```python
from build123d import *

# Parameters (mm, degrees)
SKETCH001_R  = 20
PAD_DEPTH    = 5
POCKET_DEPTH = 2.5


with BuildPart() as part:
    # Sketch001 (on DatumPlane) → Pad (new body)
    with BuildSketch(Plane.XY):
        Circle(SKETCH001_R)
    extrude(amount=-PAD_DEPTH)

    # Sketch (on DatumPlane) → Pocket (cut)
    with BuildSketch(Plane(origin=(-14.5, 14.5, 0), x_dir=(1, 0, 0), z_dir=(0, 0, 1))):
        with BuildLine():
            add(Edge.make_bspline(
                [(19.881144, 0), (19.819056, -0.000794), (19.75485, -0.003847), (19.69135, -0.008819)],
                knots=[0, 0, 0, 0, 1, 1, 1, 1], degree=3))
            add(Edge.make_bspline(
                [(19.69135, -0.008819), (17.16405, -0.4451), (15.774106, -3.117779), (15.573022, -5.474688)],
                knots=[0, 0, 0, 0, 1, 1, 1, 1], degree=3))
            add(Edge.make_bspline(
                [(15.573022, -5.474688), (15.278806, -7.61365), (16.221428, -10.361789), (18.569517, -10.841567)],
                knots=[0, 0, 0, 0, 1, 1, 1, 1], degree=3))
            add(Edge.make_bspline(
                [(18.569517, -10.841567), (18.9103, -10.906478), (19.263783, -10.876844), (19.596806, -10.786533)],
                knots=[0, 0, 0, 0, 1, 1, 1, 1], degree=3))
            add(Edge.make_bspline(
                [(19.596806, -10.786533), (22.424672, -9.838267), (23.689733, -6.489136), (23.281217, -3.715456)],
                knots=[0, 0, 0, 0, 1, 1, 1, 1], degree=3))
            add(Edge.make_bspline(
                [(23.281217, -3.715456), (23.161978, -1.923627), (21.811544, 0.024624), (19.881144, 0)],
                knots=[0, 0, 0, 0, 1, 1, 1, 1], degree=3))
        make_face()
        with BuildLine():
            add(Edge.make_bspline(
                [(9.165872, -0.114653), (7.593894, -0.153233), (6.369756, -1.747167), (6.120694, -3.245556)],
                knots=[0, 0, 0, 0, 1, 1, 1, 1], degree=3))
            add(Edge.make_bspline(
                [(6.120694, -3.245556), (5.595691, -6.21411), (6.946053, -9.902472), (10.038644, -10.841567)],
                knots=[0, 0, 0, 0, 1, 1, 1, 1], degree=3))
            add(Edge.make_bspline(
                [(10.038644, -10.841567), (10.328628, -10.904361), (10.627783, -10.910711), (10.920589, -10.865556)],
                knots=[0, 0, 0, 0, 1, 1, 1, 1], degree=3))
            add(Edge.make_bspline(
                [(10.920589, -10.865556), (13.01115, -10.517011), (13.896622, -8.173861), (13.809133, -6.281632)],
                knots=[0, 0, 0, 0, 1, 1, 1, 1], degree=3))
            add(Edge.make_bspline(
                [(13.809133, -6.281632), (13.746339, -3.785941), (12.449528, -0.900148), (9.858022, -0.198473)],
                knots=[0, 0, 0, 0, 1, 1, 1, 1], degree=3))
            add(Edge.make_bspline(
                [(9.858022, -0.198473), (9.620956, -0.135615), (9.390239, -0.109142), (9.165872, -0.114653)],
                knots=[0, 0, 0, 0, 1, 1, 1, 1], degree=3))
        make_face()
        with BuildLine():
            add(Edge.make_bspline(
                [(26.729267, -8.546042), (24.010761, -8.709025), (22.146683, -11.421886), (21.880689, -13.954831)],
                knots=[0, 0, 0, 0, 1, 1, 1, 1], degree=3))
            add(Edge.make_bspline(
                [(21.880689, -13.954831), (21.521561, -15.781514), (22.495228, -18.225558), (24.580144, -18.371608)],
                knots=[0, 0, 0, 0, 1, 1, 1, 1], degree=3))
            add(Edge.make_bspline(
                [(24.580144, -18.371608), (27.486328, -18.335625), (29.469644, -15.229769), (29.551489, -12.557125)],
                knots=[0, 0, 0, 0, 1, 1, 1, 1], degree=3))
            add(Edge.make_bspline(
                [(29.551489, -12.557125), (29.735639, -10.789708), (28.694239, -8.644114), (26.729267, -8.546042)],
                knots=[0, 0, 0, 0, 1, 1, 1, 1], degree=3))
        make_face()
        with BuildLine():
            add(Edge.make_bspline(
                [(2.932289, -9.148586), (1.775601, -9.138708), (0.638034, -9.831564), (0.260068, -11.007019)],
                knots=[0, 0, 0, 0, 1, 1, 1, 1], degree=3))
            add(Edge.make_bspline(
                [(0.260068, -11.007019), (-0.748383, -14.152386), (1.276632, -18.135953), (4.607983, -18.797058)],
                knots=[0, 0, 0, 0, 1, 1, 1, 1], degree=3))
            add(Edge.make_bspline(
                [(4.607983, -18.797058), (5.998351, -19.034831), (7.219809, -17.967325), (7.564826, -16.682508)],
                knots=[0, 0, 0, 0, 1, 1, 1, 1], degree=3))
            add(Edge.make_bspline(
                [(7.564826, -16.682508), (8.295076, -13.934369), (6.794712, -10.743847), (4.255206, -9.496425)],
                knots=[0, 0, 0, 0, 1, 1, 1, 1], degree=3))
            add(Edge.make_bspline(
                [(4.255206, -9.496425), (3.841538, -9.264297), (3.384973, -9.152114), (2.932289, -9.148586)],
                knots=[0, 0, 0, 0, 1, 1, 1, 1], degree=3))
        make_face()
        with BuildLine():
            add(Edge.make_bspline(
                [(15.120761, -14.788092), (12.853106, -14.793031), (10.550172, -15.943792), (9.081911, -17.656881)],
                knots=[0, 0, 0, 0, 1, 1, 1, 1], degree=3))
            add(Edge.make_bspline(
                [(9.081911, -17.656881), (7.495822, -19.653603), (6.196753, -21.976997), (5.688542, -24.496536)],
                knots=[0, 0, 0, 0, 1, 1, 1, 1], degree=3))
            add(Edge.make_bspline(
                [(5.688542, -24.496536), (5.07111, -26.309814), (6.470509, -28.397553), (8.409517, -28.410253)],
                knots=[0, 0, 0, 0, 1, 1, 1, 1], degree=3))
            add(Edge.make_bspline(
                [(8.409517, -28.410253), (10.742083, -28.474458), (12.746567, -26.872847), (15.065728, -26.754314)],
                knots=[0, 0, 0, 0, 1, 1, 1, 1], degree=3))
            add(Edge.make_bspline(
                [(15.065728, -26.754314), (17.033522, -26.454453), (18.795294, -27.477508), (20.564828, -28.147786)],
                knots=[0, 0, 0, 0, 1, 1, 1, 1], degree=3))
            add(Edge.make_bspline(
                [(20.564828, -28.147786), (22.071189, -28.791958), (24.152578, -28.545014), (24.921633, -26.923647)],
                knots=[0, 0, 0, 0, 1, 1, 1, 1], degree=3))
            add(Edge.make_bspline(
                [(24.921633, -26.923647), (25.526294, -25.271942), (24.635883, -23.509464), (23.898578, -22.042614)],
                knots=[0, 0, 0, 0, 1, 1, 1, 1], degree=3))
            add(Edge.make_bspline(
                [(23.898578, -22.042614), (22.394333, -19.660658), (20.782139, -17.157347), (18.315517, -15.670036)],
                knots=[0, 0, 0, 0, 1, 1, 1, 1], degree=3))
            add(Edge.make_bspline(
                [(18.315517, -15.670036), (17.327033, -15.057614), (16.228483, -14.785975), (15.120761, -14.788092)],
                knots=[0, 0, 0, 0, 1, 1, 1, 1], degree=3))
        make_face()
    extrude(amount=-POCKET_DEPTH, mode=Mode.SUBTRACT)


solid = part.part
```
Model file for the job. Use its own axes, mm. A direction names the side the tool comes from. Give positions to 0.01 mm unless a question says otherwise; leave off trailing zeros. Order: outer loops, then holes, each group sorted by start corner. A loop starts at its lowest first (then second) coordinate and runs counter-clockwise, first axis right, second up.
1) Saw through at D-D, the plane y = 15. Write the cut outline in (x, z).
2) Saw through at B-B, the plane z = -1.35. Count the separate pieces of the cut face and the enclosed holes in it, then the cut area to 3 significant figures.
3) Mould opens along Y. For faces 3 (the flat face through (0, 0, -5)), 4 (the cylindrical face through (-4.336, -19.524, -2.465)), 5 (the flat face through (5, 9, -2.5)) say: +Y half, -Y half, draft (parallel to the pull), parting line (faces both ways), or undercut.
4) 3-axis set-ups, long thin cutter, end or side, ignore diameter. For faces 1 (the flat face through (1, -7, -2.5)), 2 (the flat face through (0, 0, 0)): which of +Z, -Z, +X, -X, +Y, -Y reach the whole face in a straight line?
5) Saw through at C-C, the plane x = 17.5. Write the cut outline in (y, z), then the cut area to 3 significant figures.
6) Saw through at A-A, the plane z = -3.8. Write the cut outline in (x, y).
7) Wall check: probe 1 along X at (y, z) = (13, -1.95); probe 2 along X at (y, z) = (8.5, -2); probe 3 along X at (y, z) = (5.5, -0.3). Give the ranges that are in metal, low to high.
8) Pin check, flat tips, straight feed: pin 1 (2 mm diameter, centred on x = -0.5, z = -3, fed in from -Y); pin 2 (4 mm diameter, centred on x = -4, y = 9.5, fed in from +Z). Stop position of each tip, or through.
Computed:
1. outline: (-13.23, -5) - (13.23, -5) - (13.23, 0) - (-13.23, 0) - close
2. separate pieces: 1
2. enclosed holes: 5
2. area: 817 mm2
3. face 3: draft
3. face 4: parting line
3. face 5: undercut
4. face 1: +Z
4. face 2: +Z, +X, -X, +Y, -Y
5. outline: (-9.68, -5) - (9.68, -5) - (9.68, 0) - (-9.68, 0) - close
5. area: 96.8 mm2
6. outline: circle Ø40 at (0, 0)
7. probe 1: x = -15.2 to -7.65, -2.51 to 2.66, 8.01 to 15.2
7. probe 2: x = -18.1 to -8.35, -0.7 to 1.03, 8.75 to 18.1
7. probe 3: x = -19.23 to -7.06, -1.24 to 1.69, 7.51 to 10.56, 13.58 to 19.23
8. pin 1: stops at y = -20
8. pin 2: stops at z = -2.5
